Part model, mm, in its own coordinate system. Face numbers are marked on the shaded views. A direction names the side the tool comes from. Coordinates: 2 decimals unless noted, no trailing zeros. Write each loop counter-clockwise with the first axis right and the second up, starting at its lowest first coordinate (ties: lowest second). Pieces come first, ordered by that corner, then holes. Notation, with made-up numbers: (14.25, 39) -> (39.25, 39) arc R25 ccw to (39.25, 55) -> close; hole circle Ø6 at (6, -36.5). An arc over 180 degrees is marked (long way). Write item = value, one per line. Start each with the question number.
Q1. Band-saw the part on B-B, the plane x = 12. List the corners of the cut face in (y, z).
Q2. Tool access for the marked faces 5, 6, 7 and 8: list every direction of +Z, -Z, +X, -X, +Y, -Y with a clear straight run to the whole face (end or side of a thin tool).
Q3. Pull direction X, two halves, no side cores. Call the marked faces 1, 2, 3 and 4: released by +X, released by -X, zero draft, split by the parting line, or undercut.
Q4. Probe line 1 (Y direction, x = 21, z = -1.75); line 2 (X direction, y = 0.5, z = -4.25); line 3 (Y direction, x = 0, z = -3.9). List the from-to ranges inside material, lowest first.
Q5. Pin check, flat tips, straight feed: P1, Ø5, axis at x = 7.5, y = -0.5, coming from the +Z side; P2, Ø5, axis at x = 0, y = 0, coming from the -Z side; P3, Ø1.3, axis at y = -4, z = -1, coming from the -X side; P4, Ø3, axis at x = -1, y = 1, coming from the +Z side. Stop position of each tip, or through.
Q6. Band-saw the part on D-D, the plane x = 23.5. List the corners of the cut face in (y, z).
Q7. Band-saw the part on A-A, the plane z = -1. List the corners of the cut face in (x, y).
Q8. Band-saw the part on C-C, the plane z = -3.5. List the corners of the cut face in (x, y), plus the area to 3 significant figures.
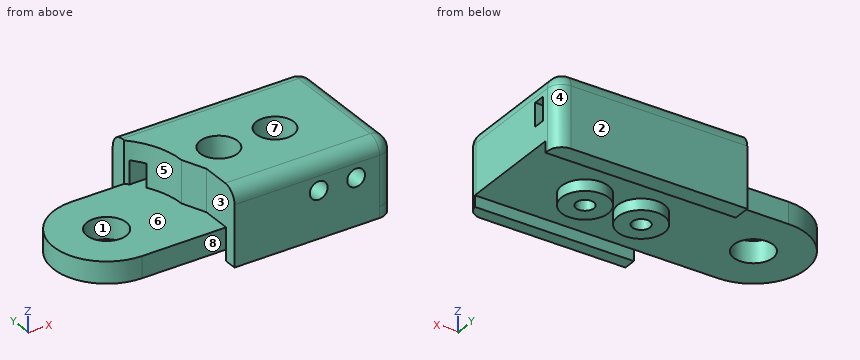
from build123d import *

# Parameters (mm, degrees)
BOSS_EXTRUDE1_DEPTH = 2
BOSS_EXTRUDE2_START = 2.5
BOSS_EXTRUDE2_DEPTH = 2.5
CUT_EXTRUDE1_DEPTH  = 2.5
BOSS_EXTRUDE3_DEPTH = 2.3
SKETCH9_R           = 2.1
CUT_EXTRUDE2_DEPTH  = 2.5
SKETCH10_R          = 2.5
BOSS_EXTRUDE4_DEPTH = 1.2
SKETCH11_R          = 0.95
CUT_EXTRUDE3_DEPTH  = 9.2
SKETCH12_R          = 2
CUT_EXTRUDE4_DEPTH  = 2.5
SKETCH14_W          = 20.343145751
SKETCH14_H          = 1.841510486
SKETCH14_W_2        = 17
SKETCH14_H_2        = 1.34163614
BOSS_EXTRUDE5_DEPTH = 1.2
FILLET1_R           = 1.5
SKETCH17_R          = 0.95
CUT_EXTRUDE5_DEPTH  = 3


# Read off the part's stored shape, not the designer's step: Boss-Extrude3
with BuildPart() as part:
    # Sketch5 → Boss-Extrude1 (new body)
    with BuildSketch(Plane.XY):
        with BuildLine():
            Line((8, 0), (9, -2.501635265))
            Line((9, -2.501635265), (9, -7.001635265))
            Line((9, -7.001635265), (26, -7.001635265))
            Line((26, -7.001635265), (26, 7.498364735))
            Line((26, 7.498364735), (5.656854249, 7.498364735))
            Line((5.656854249, 7.498364735), (5.656854249, 5.656854249))
            ThreePointArc((5.656854249, 5.656854249), (7.39103626, 3.061467459), (8, 0))
        make_face()
    extrude(amount=BOSS_EXTRUDE1_DEPTH)

    # Sketch6 → Boss-Extrude2 (add)
    with BuildSketch(Plane(origin=(0, 0, 0), x_dir=(-1, 0, 0), z_dir=(0, 0, -1)).offset(BOSS_EXTRUDE2_START)):
        with BuildLine():
            Line((-5.656854249, 7.498364735), (-5.656854249, 5.656854249))
            ThreePointArc((-5.656854249, 5.656854249), (-7.39103626, 3.061467459), (-8, 0))
            Line((-8, 0), (-9, -2.501635265))
            Line((-9, -2.501635265), (-9, -7.001635265))
            Line((-9, -7.001635265), (-26, -7.001635265))
            Line((-26, -7.001635265), (-26, 7.498364735))
            Line((-26, 7.498364735), (-5.656854249, 7.498364735))
        make_face()
    extrude(amount=-BOSS_EXTRUDE2_DEPTH)

    # Sketch7 → Cut-Extrude1 (cut)
    with BuildSketch(Plane(origin=(0, 0, -2.5), x_dir=(-1, 0, 0), z_dir=(0, 0, -1))):
        Polygon((-26, 5.298364735), (-2.738141148, 5.298364735), (-2.738141148, 3.998364735), (-29.849535112, 3.998364735), (-29.849535112, 5.298364735), align=None)
    extrude(amount=-CUT_EXTRUDE1_DEPTH, mode=Mode.SUBTRACT)

    # Boss-Extrude3 outline → Boss-Extrude3 (add)
    with BuildSketch(Plane(origin=(0, 0, -2.5), x_dir=(-1, 0, 0), z_dir=(0, 0, -1))):
        with BuildLine():
            Line((-9, -7.001635265), (-9, -5.659999125))
            Line((-9, -5.659999125), (0, -5.659998688))
            ThreePointArc((0, -5.659998688), (5.659998688, 0), (0, 5.659998688))
            Line((0, 5.659998688), (-5.656854249, 5.656854249))
            Line((-5.656854249, 5.656854249), (-5.656854249, 7.498364735))
            Line((-5.656854249, 7.498364735), (-26, 7.498364735))
            Line((-26, 7.498364735), (-26, -7.001635265))
            Line((-26, -7.001635265), (-9, -7.001635265))
        make_face()
    extrude(amount=BOSS_EXTRUDE3_DEPTH)

    # Sketch9 → Cut-Extrude2 (cut)
    with BuildSketch(Plane(origin=(0, 0, -4.8), x_dir=(-1, 0, 0), z_dir=(0, 0, -1))):
        Circle(SKETCH9_R)
    extrude(amount=-CUT_EXTRUDE2_DEPTH, mode=Mode.SUBTRACT)

    # Sketch10 → Boss-Extrude4 (add)
    with BuildSketch(Plane(origin=(0, 0, -4.8), x_dir=(-1, 0, 0), z_dir=(0, 0, -1))):
        with Locations((-12, 0)):
            Circle(SKETCH10_R)
        with Locations((-18, 0)):
            Circle(SKETCH10_R)
    extrude(amount=BOSS_EXTRUDE4_DEPTH)

    # Sketch11 → Cut-Extrude3 (cut)
    with BuildSketch(Plane(origin=(0, 0, -6), x_dir=(-1, 0, 0), z_dir=(0, 0, -1))):
        with Locations((-18, 0)):
            Circle(SKETCH11_R)
        with Locations((-12, 0)):
            Circle(SKETCH11_R)
    extrude(amount=-CUT_EXTRUDE3_DEPTH, mode=Mode.SUBTRACT)

    # Sketch12 → Cut-Extrude4 (cut)
    with BuildSketch(Plane.XY.offset(2)):
        with Locations((12, 0)):
            Circle(SKETCH12_R)
        with Locations((18, 0)):
            Circle(SKETCH12_R)
    extrude(amount=-CUT_EXTRUDE4_DEPTH, mode=Mode.SUBTRACT)

    # Sketch14 → Boss-Extrude5 (add)
    with BuildSketch(Plane(origin=(0, 0, -4.8), x_dir=(-1, 0, 0), z_dir=(0, 0, -1))):
        with Locations((-15.828427124, 6.577609492)):
            Rectangle(SKETCH14_W, SKETCH14_H)
        with Locations((-17.5, -6.330817195)):
            Rectangle(SKETCH14_W_2, SKETCH14_H_2)
    extrude(amount=BOSS_EXTRUDE5_DEPTH)

    # Fillet1
    # the kernel refuses this fillet: 1.5 mm, written as the material it takes off along each edge
    with BuildSketch(Plane(origin=(24.5, -5.501635265, 0.5), x_dir=(0, 0, 1), z_dir=(0, -1, 0))) as fillet1_piece_1_section:
        Polygon((0, 0), (FILLET1_R, 0), (FILLET1_R, -FILLET1_R), (0, -FILLET1_R), align=None)
    fillet1_piece_1 = extrude(amount=FILLET1_R, mode=Mode.PRIVATE)
    fillet1_piece_1 = fillet1_piece_1 - Plane(origin=(24.5, -5.501635265, 0.5), x_dir=(-0.7071067811865475, 0, -0.7071067811865475), z_dir=(0, -1, 0)) * Sphere(FILLET1_R, mode=Mode.PRIVATE)
    add(fillet1_piece_1, mode=Mode.SUBTRACT)
    with BuildSketch(Plane(origin=(24.5, 5.998364735, 0.5), x_dir=(0, 0, 1), z_dir=(0, 1, 0))) as fillet1_piece_2_section:
        Polygon((0, 0), (FILLET1_R, 0), (FILLET1_R, FILLET1_R), (0, FILLET1_R), align=None)
    fillet1_piece_2 = extrude(amount=FILLET1_R, mode=Mode.PRIVATE)
    fillet1_piece_2 = fillet1_piece_2 - Plane(origin=(24.5, 5.998364735, 0.5), x_dir=(-0.7071067811865475, 0, -0.7071067811865475), z_dir=(0, 1, 0)) * Sphere(FILLET1_R, mode=Mode.PRIVATE)
    add(fillet1_piece_2, mode=Mode.SUBTRACT)
    with BuildSketch(Plane(origin=(26, -5.501635265, 2), x_dir=(-1, 0, 0), z_dir=(0, 1, 0))) as fillet1_piece_3:
        with BuildLine():
            CenterArc((FILLET1_R, -FILLET1_R), FILLET1_R, 90, 90)
            Line((0, -FILLET1_R), (0, 0))
            Line((0, 0), (FILLET1_R, 0))
        make_face()
    extrude(amount=11.5, mode=Mode.SUBTRACT)
    with BuildSketch(Plane(origin=(26, -7.001635265, -2.5), x_dir=(-1, 0, 0), z_dir=(0, 0, 1))) as fillet1_piece_4:
        with BuildLine():
            CenterArc((FILLET1_R, -FILLET1_R), FILLET1_R, 90, 90)
            Line((0, -FILLET1_R), (0, 0))
            Line((0, 0), (FILLET1_R, 0))
        make_face()
    extrude(amount=3, mode=Mode.SUBTRACT)
    with BuildSketch(Plane(origin=(5.25, -7.001635265, 2), x_dir=(0, 1, 0), z_dir=(1, 0, 0))) as fillet1_piece_5:
        with BuildLine():
            CenterArc((FILLET1_R, -FILLET1_R), FILLET1_R, 90, 90)
            Line((0, -FILLET1_R), (0, 0))
            Line((0, 0), (FILLET1_R, 0))
        make_face()
    extrude(amount=19.25, mode=Mode.SUBTRACT)
    with BuildSketch(Plane(origin=(24.5, 7.498364735, 2), x_dir=(0, -1, 0), z_dir=(-1, 0, 0))) as fillet1_piece_6:
        with BuildLine():
            CenterArc((FILLET1_R, -FILLET1_R), FILLET1_R, 90, 90)
            Line((0, -FILLET1_R), (0, 0))
            Line((0, 0), (FILLET1_R, 0))
        make_face()
    extrude(amount=22.593145751, mode=Mode.SUBTRACT)
    with BuildSketch(Plane(origin=(26, 7.498364735, -2.5), x_dir=(-1, 0, 0), z_dir=(0, 0, 1))) as fillet1_piece_7:
        with BuildLine():
            CenterArc((FILLET1_R, FILLET1_R), FILLET1_R, 180, 90)
            Line((0, FILLET1_R), (0, 0))
            Line((0, 0), (FILLET1_R, 0))
        make_face()
    extrude(amount=3, mode=Mode.SUBTRACT)
    with BuildSketch(Plane(origin=(26, 7.498364735, -2.5), x_dir=(-1.0, -1.9174232572065026e-10, 0), z_dir=(0, 0, -1))) as fillet1_piece_8:
        with BuildLine():
            CenterArc((FILLET1_R, -FILLET1_R), FILLET1_R, 90.000000011, 90)
            Line((FILLET1_R * 1.9173522033e-10, -FILLET1_R), (0, 0))
            Line((0, 0), (FILLET1_R, 0))
        make_face()
    extrude(amount=2.3, mode=Mode.SUBTRACT)
    with BuildSketch(Plane(origin=(26, 7.498364735, -4.8), x_dir=(-1, 0, 0), z_dir=(0, 0, -1))) as fillet1_piece_9:
        with BuildLine():
            CenterArc((FILLET1_R, -FILLET1_R), FILLET1_R, 90, 90)
            Line((0, -FILLET1_R), (0, 0))
            Line((0, 0), (FILLET1_R, 0))
        make_face()
    extrude(amount=4.95, mode=Mode.SUBTRACT)
    with BuildSketch(Plane(origin=(26, -7.001635265, -2.5), x_dir=(-1.0, -1.9169850891861218e-10, 0), z_dir=(0, 0, -1))) as fillet1_piece_10:
        with BuildLine():
            CenterArc((FILLET1_R, FILLET1_R), FILLET1_R, 180.000000011, 90)
            Line((-FILLET1_R * 1.91707982785e-10, FILLET1_R), (0, 0))
            Line((0, 0), (FILLET1_R, 0))
        make_face()
    extrude(amount=2.3, mode=Mode.SUBTRACT)
    with BuildSketch(Plane(origin=(26, -7.001635265, -4.8), x_dir=(-1, 0, 0), z_dir=(0, 0, -1))) as fillet1_piece_11:
        with BuildLine():
            CenterArc((FILLET1_R, FILLET1_R), FILLET1_R, 180, 90)
            Line((0, FILLET1_R), (0, 0))
            Line((0, 0), (FILLET1_R, 0))
        make_face()
    extrude(amount=4.95, mode=Mode.SUBTRACT)

    # Sketch17 → Cut-Extrude5 (cut)
    with BuildSketch(Plane.XZ.offset(7.001635265)):
        with Locations((22, -1)):
            Circle(SKETCH17_R)
        with Locations((18, -1)):
            Circle(SKETCH17_R)
    extrude(amount=-CUT_EXTRUDE5_DEPTH, mode=Mode.SUBTRACT)


solid = part.part
Ans:
q1.outline = (-7, -6) -> (-5.66, -6) -> (-5.66, -4.8) -> (-2.5, -4.8) -> (-2.5, -6) -> (-0.95, -6) -> (-0.95, -0.5) -> (-2, -0.5) -> (-2, 2) -> (-5.5, 2) arc R1.5 ccw to (-7, 0.5) -> close; (0.95, -6) -> (2.5, -6) -> (2.5, -4.8) -> (5.66, -4.8) -> (5.66, -6) -> (7.5, -6) -> (7.5, 0.5) arc R1.5 ccw to (6, 2) -> (2, 2) -> (2, -0.5) -> (0.95, -0.5) -> close; hole (4, -2.5) -> (5.3, -2.5) -> (5.3, 0) -> (4, 0) -> close
q2.face_5 = +Z, -X, -Y
q2.face_6 = -X
q2.face_7 = +Z
q2.face_8 = +Z, -Z, -X, -Y
q3.face_1 = undercut
q3.face_2 = zero draft
q3.face_3 = released by -X
q3.face_4 = released by +X
q4.line_1 = -7 to 4, 5.3 to 7.5
q4.line_2 = -5.64 to -2.04, 2.04 to 11.19, 12.81 to 17.19, 18.81 to 26
q4.line_3 = -5.66 to -2.1, 2.1 to 5.66
q5.P1 = 2
q5.P2 = -4.8
q5.P3 = 9
q5.P4 = -2.5
q6.outline = (-7, -6) -> (-5.66, -6) -> (-5.66, -4.8) -> (5.66, -4.8) -> (5.66, -6) -> (7.5, -6) -> (7.5, 0.5) arc R1.5 ccw to (6, 2) -> (-5.5, 2) arc R1.5 ccw to (-7, 0.5) -> close; hole (4, -2.5) -> (5.3, -2.5) -> (5.3, 0) -> (4, 0) -> close
q7.outline = (5.66, 5.66) arc R8 cw to (5.99, 5.3) -> (26, 5.3) -> (26, 6) arc R1.5 ccw to (24.5, 7.5) -> (5.66, 7.5) -> close; (6.93, 4) arc R8 cw to (8, 0) -> (9, -2.5) -> (9, -7) -> (17.05, -7) -> (17.05, -4) -> (18.95, -4) -> (18.95, -7) -> (21.05, -7) -> (21.05, -4) -> (22.95, -4) -> (22.95, -7) -> (24.5, -7) arc R1.5 ccw to (26, -5.5) -> (26, 4) -> close; hole circle Ø1.9 at (12, 0); hole circle Ø1.9 at (18, 0)
q8.outline = (0, -5.66) -> (9, -5.66) -> (9, -7) -> (24.5, -7) arc R1.5 ccw to (26, -5.5) -> (26, 6) arc R1.5 ccw to (24.5, 7.5) -> (5.66, 7.5) -> (5.66, 5.66) -> (0, 5.66) arc R5.66 ccw to start; hole circle Ø4.2 at (0, 0); hole circle Ø1.9 at (12, 0); hole circle Ø1.9 at (18, 0)
q8.area = 384 mm2
